from build123d import *

# Parameters (mm, degrees)
SKETCH003_W     = 170
SKETCH003_H     = 90
SKETCH003_W_2   = 160
SKETCH003_H_2   = 80
PAD_DEPTH       = 3
PAD001_DEPTH    = 3
PAD002_DEPTH    = 3
PAD003_DEPTH    = 3
PAD004_DEPTH    = 3
PAD005_DEPTH    = 10
PAD006_DEPTH    = 10
PAD007_DEPTH    = 24
SKETCH014_R     = 1.65
HOLE_DEPTH      = 30
SKETCH015_R     = 1.325
HOLE001_DEPTH   = 30
SKETCH016_R     = 1.325
HOLE002_DEPTH   = 30
SKETCH017_R     = 1.325
HOLE003_DEPTH   = 30
FILLET_R        = 0.3
FILLET001_R     = 0.3
FILLET002_R     = 0.3
FILLET003_R     = 0.3
FILLET004_R     = 0.3
FILLET005_R     = 0.3
FILLET006_R     = 0.3
FILLET007_R     = 0.3
FILLET008_R     = 0.3
FILLET009_R     = 0.3
SKETCH018_W     = 3.707428
SKETCH018_H     = 3.707435
PAD008_DEPTH    = 27
SKETCH019_W     = 4.325348
SKETCH019_H     = 3.769226
PAD009_DEPTH    = 27
SKETCH020_W     = 4.473305
SKETCH020_H     = 4.349049
PAD010_DEPTH    = 27
SKETCH021_W     = 3.413819
SKETCH021_H     = 3.638272
PAD011_DEPTH    = 27
SKETCH023_R     = 1.4
POCKET_DEPTH    = 30
SKETCH024_R     = 1.4
POCKET001_DEPTH = 30
SKETCH025_R     = 1.4
POCKET002_DEPTH = 30
SKETCH026_R     = 1.4
POCKET003_DEPTH = 30
SKETCH027_R     = 1.5
POCKET004_DEPTH = 5
CHAMFER_SIZE    = 1


with BuildPart() as part:
    # Sketch003 → Pad (new body)
    with BuildSketch(Plane.XY):
        Rectangle(SKETCH003_W, SKETCH003_H)
        Rectangle(SKETCH003_W_2, SKETCH003_H_2, mode=Mode.SUBTRACT)
    extrude(amount=PAD_DEPTH)

    # Sketch005 → Pad001 (join)
    with BuildSketch(Plane.XY):
        Polygon((-70, 45), (-75, 50), (-120, 50), (-120, 40), (-85, 5), (-85, 12), (-113, 40), (-95, 40), (-85, 30), (-85, 45), align=None)
    extrude(amount=PAD001_DEPTH)

    # Sketch007 → Pad002 (join)
    with BuildSketch(Plane.XY):
        Polygon((70, 45), (75, 50), (120, 50), (120, 40), (85, 5), (85, 12), (113, 40), (95, 40), (85, 30), (85, 45), align=None)
    extrude(amount=PAD002_DEPTH)

    # Sketch008 → Pad003 (join)
    with BuildSketch(Plane.XY):
        Polygon((70, -45), (75, -50), (120, -50), (120, -40), (85, -5), (85, -12), (113, -40), (95, -40), (85, -30), (85, -45), align=None)
    extrude(amount=PAD003_DEPTH)

    # Sketch009 → Pad004 (join)
    with BuildSketch(Plane.XY):
        Polygon((-70, -45), (-75, -50), (-115, -90), (-90, -115), (-90, -120), (-120, -120), (-120, -50), (-120, -40), (-85, -5), (-85, -12), (-113, -40), (-95, -40), (-85, -30), (-85, -45), align=None)
        Polygon((-115, -50), (-115, -83), (-82, -50), align=None, mode=Mode.SUBTRACT)
        Polygon((-115, -97), (-115, -115), (-97, -115), align=None, mode=Mode.SUBTRACT)
    extrude(amount=PAD004_DEPTH)

    # Sketch011 (on Face23 of Pad004) → Pad005 (join)
    with BuildSketch(Plane.XY.offset(3)):
        Polygon((-120, 50), (-120, 40), (-117, 40), (-117, 47), (-110, 47), (-110, 50), align=None)
    extrude(amount=PAD005_DEPTH)

    # Sketch012 (on Face22 of Pad005) → Pad006 (join)
    with BuildSketch(Plane.XY.offset(3)):
        Polygon((120, 50), (110, 50), (110, 47), (117, 47), (117, 40), (120, 40), align=None)
    extrude(amount=PAD006_DEPTH)

    # Sketch013 (on Face4 of Pad006) → Pad007 (join)
    with BuildSketch(Plane.XY.offset(3)):
        Polygon((-85, 45), (-85, 30), (-80, 30), (-80, 40), (-70, 40), (-70, 45), align=None)
        Polygon((85, 45), (85, 30), (80, 30), (80, 40), (70, 40), (70, 45), align=None)
        Polygon((85, -45), (85, -30), (80, -30), (80, -40), (70, -40), (70, -45), align=None)
        Polygon((-85, -45), (-85, -30), (-80, -30), (-80, -40), (-70, -40), (-70, -45), align=None)
    extrude(amount=PAD007_DEPTH)

    # Sketch014 (on Face80 of Pad007) → Hole (cut)
    with BuildSketch(Plane.XY.offset(27)):
        with Locations((-82.5, 42.5)):
            Circle(SKETCH014_R)
    extrude(amount=-HOLE_DEPTH, mode=Mode.SUBTRACT)

    # Sketch015 (on Face99 of Hole) → Hole001 (cut)
    with BuildSketch(Plane.XY.offset(27)):
        with Locations((-82.5, -42.5)):
            Circle(SKETCH015_R)
    extrude(amount=-HOLE001_DEPTH, mode=Mode.SUBTRACT)

    # Sketch016 (on Face84 of Hole001) → Hole002 (cut)
    with BuildSketch(Plane.XY.offset(27)):
        with Locations((82.5, 42.5)):
            Circle(SKETCH016_R)
    extrude(amount=-HOLE002_DEPTH, mode=Mode.SUBTRACT)

    # Sketch017 (on Face104 of Hole002) → Hole003 (cut)
    with BuildSketch(Plane.XY.offset(27)):
        with Locations((82.5, -42.5)):
            Circle(SKETCH017_R)
    extrude(amount=-HOLE003_DEPTH, mode=Mode.SUBTRACT)

    # Fillet
    fillet_edges = [part.edges().sort_by_distance(p)[0] for p in [
        (-115, -97, 1.5),
    ]]
    fillet(fillet_edges, radius=FILLET_R)

    # Fillet001
    fillet001_edges = [part.edges().sort_by_distance(p)[0] for p in [
        (-115, -115, 1.5),
    ]]
    fillet(fillet001_edges, radius=FILLET001_R)

    # Fillet002
    fillet002_edges = [part.edges().sort_by_distance(p)[0] for p in [
        (-97, -115, 1.5),
    ]]
    fillet(fillet002_edges, radius=FILLET002_R)

    # Fillet003
    fillet003_edges = [part.edges().sort_by_distance(p)[0] for p in [
        (-115, -90, 1.5),
    ]]
    fillet(fillet003_edges, radius=FILLET003_R)

    # Fillet004
    fillet004_edges = [part.edges().sort_by_distance(p)[0] for p in [
        (-115, -50, 1.5),
        (-115, -83, 1.5),
        (-82, -50, 1.5),
    ]]
    fillet(fillet004_edges, radius=FILLET004_R)

    # Fillet005
    fillet005_edges = [part.edges().sort_by_distance(p)[0] for p in [
        (-95, -40, 1.5),
        (-85, -12, 1.5),
        (-113, -40, 1.5),
    ]]
    fillet(fillet005_edges, radius=FILLET005_R)

    # Fillet006
    fillet006_edges = [part.edges().sort_by_distance(p)[0] for p in [
        (-117, 43.5, 3),
        (-113.5, 47, 3),
    ]]
    fillet(fillet006_edges, radius=FILLET006_R)

    # Fillet007
    fillet007_edges = [part.edges().sort_by_distance(p)[0] for p in [
        (-113, 40, 1.5),
        (-85, 12, 1.5),
    ]]
    fillet(fillet007_edges, radius=FILLET007_R)

    # Fillet008
    fillet008_edges = [part.edges().sort_by_distance(p)[0] for p in [
        (113.5, 47, 3),
        (117, 43.5, 3),
        (113, 40, 1.5),
        (85, 12, 1.5),
    ]]
    fillet(fillet008_edges, radius=FILLET008_R)

    # Fillet009
    fillet009_edges = [part.edges().sort_by_distance(p)[0] for p in [
        (113, -40, 1.5),
        (85, -12, 1.5),
    ]]
    fillet(fillet009_edges, radius=FILLET009_R)

    # Sketch018 (on Face81 of Fillet009) → Pad008 (join)
    with BuildSketch(Plane.XY.offset(27)):
        with Locations((82.542801, -42.437325)):
            Rectangle(SKETCH018_W, SKETCH018_H)
    extrude(amount=-PAD008_DEPTH)

    # Sketch019 (on Face37 of Pad008) → Pad009 (join)
    with BuildSketch(Plane.XY.offset(27)):
        with Locations((82.440964, 42.612553)):
            Rectangle(SKETCH019_W, SKETCH019_H)
    extrude(amount=-PAD009_DEPTH)

    # Sketch020 (on Face85 of Pad009) → Pad010 (join)
    with BuildSketch(Plane.XY.offset(27)):
        with Locations((-82.434589, 42.41842)):
            Rectangle(SKETCH020_W, SKETCH020_H)
    extrude(amount=-PAD010_DEPTH)

    # Sketch021 (on Face18 of Pad010) → Pad011 (join)
    with BuildSketch(Plane.XY.offset(27)):
        with Locations((-82.443809, -42.548483)):
            Rectangle(SKETCH021_W, SKETCH021_H)
    extrude(amount=-PAD011_DEPTH)

    # Sketch023 (on Face83 of Pad011) → Pocket (cut)
    with BuildSketch(Plane.XY.offset(27)):
        with Locations((-82.5, 42.5)):
            Circle(SKETCH023_R)
    extrude(amount=-POCKET_DEPTH, mode=Mode.SUBTRACT)

    # Sketch024 (on Face99 of Hole) → Pocket001 (cut)
    with BuildSketch(Plane.XY.offset(27)):
        with Locations((-82.5, -42.5)):
            Circle(SKETCH024_R)
    extrude(amount=-POCKET001_DEPTH, mode=Mode.SUBTRACT)

    # Sketch025 (on Face84 of Hole001) → Pocket002 (cut)
    with BuildSketch(Plane.XY.offset(27)):
        with Locations((82.5, 42.5)):
            Circle(SKETCH025_R)
    extrude(amount=-POCKET002_DEPTH, mode=Mode.SUBTRACT)

    # Sketch026 (on Face104 of Hole002) → Pocket003 (cut)
    with BuildSketch(Plane.XY.offset(27)):
        with Locations((82.5, -42.5)):
            Circle(SKETCH026_R)
    extrude(amount=-POCKET003_DEPTH, mode=Mode.SUBTRACT)

    # Sketch027 (on Face6 of Pocket003) → Pocket004 (cut)
    with BuildSketch(Plane.XY.offset(3)):
        with Locations((-115, -45)):
            Circle(SKETCH027_R)
        with Locations((115, -45)):
            Circle(SKETCH027_R)
    extrude(amount=-POCKET004_DEPTH, mode=Mode.SUBTRACT)

    # Chamfer
    chamfer_edges = [part.edges().sort_by_distance(p)[0] for p in [
        (-116.5, -45, 3),
        (113.5, -45, 3),
    ]]
    chamfer(chamfer_edges, length=CHAMFER_SIZE)


solid = part.part
Input: part model. Units: mm. Frame: model coordinates. A direction names the side the tool comes from. Coordinates: 2 decimals unless noted, no trailing zeros. Loops run counter-clockwise (first coordinate to the right, second up) from the corner with the lowest first, then second, coordinate; pieces in that order, holes last. Notation, with made-up numbers: (46, 32) - (57, 32) arc R25 cw to (57, 48) - close; hole circle Ø3 at (74, -29). An arc over 180 degrees is marked (long way). Answer in a Markdown table with one row per item. Add a question column.
Item 1: Access query for faces 1 (the flat face through (-70, -42, 15)), 2 (the flat face through (83, -30, 15)), 3 (the flat face through (117, 44, 8)), 4 (the flat face through (-103, 23, 1)), 5 (the flat face through (90, 35, 1)). Directions: +Z, -Z, +X, -X, +Y, -Y. A direction counts if a zero-diameter tool reaches every point of the face in a straight line with its end or side. Return the directions, or none.
Item 2: Section query A-A on z = 20.25. Return the cut outline in (x, y).
Item 3: Contact query for flat-ended pins moving along their axis: P1, Ø1.5, axis at x = 103.5, z = 1, coming from the -Y side; P2, Ø4, axis at x = -81.5, z = 13, coming from the +Y side; P3, Ø8, axis at y = -2, z = 9, coming from the +X side; P4, Ø1.5, axis at y = -70, z = 2, coming from the +X side. Output: stop coordinate, or through.
Item 4: Section query B-B on y = -77.5. Return the cut outline in (x, z).
Item 5: Line query: line 1 along Y through (x, z) = (82.5, 17); line 2 along X through (y, z) = (32, 2.25); line 3 along X through (y, z) = (37.5, 22). Output: solid intervals per line, ascending. Write a range as [from, to].
Item 6: Mould query, pull axis X, two halves, no side actions, for faces 6 (the flat face through (-103, -23, 1)), 7 (the flat face through (116, 47.3, 13)), 8 (the flat face through (-99, -26, 1)), 9 (the flat face through (85, -38, 15)). Classes: released by +X, released by -X, zero draft, split by the parting line, or undercut.
Recorded:
| question | item | result |
|---|---|---|
| 1 | face 1 | +Z, +Y, -Y |
| 1 | face 2 | +Z, +X, -X |
| 1 | face 3 | +Z, -Y |
| 1 | face 4 | +Z, -Z, -X |
| 1 | face 5 | +Z, -Z |
| 2 | outline | (-85, -45) - (-70, -45) - (-70, -40) - (-80, -40) - (-80, -30) - (-85, -30) - close; (-85, 30) - (-80, 30) - (-80, 40) - (-70, 40) - (-70, 45) - (-85, 45) - close; (70, -45) - (85, -45) - (85, -30) - (80, -30) - (80, -40) - (70, -40) - close; (70, 40) - (80, 40) - (80, 30) - (85, 30) - (85, 45) - (70, 45) - close; hole circle Ø2.8 at (-82.5, -42.5); hole circle Ø2.8 at (-82.5, 42.5); hole circle Ø2.8 at (82.5, -42.5); hole circle Ø2.8 at (82.5, 42.5) |
| 3 | P1 | y = -50 |
| 3 | P2 | y = 45 |
| 3 | P3 | through |
| 3 | P4 | x = -94.25 |
| 4 | outline | (-120, 0) - (-115, 0) - (-115, 3) - (-120, 3) - close; (-109.5, 0) - (-102.5, 0) - (-102.5, 3) - (-109.5, 3) - close |
| 5 | line 1 | [-45, -43.9], [-41.1, -30], [30, 41.1], [43.9, 45] |
| 5 | line 2 | [-112, -105], [-87, -80], [80, 87], [105, 112] |
| 5 | line 3 | [-85, -80], [80, 85] |
| 6 | face 6 | released by -X |
| 6 | face 7 | zero draft |
| 6 | face 8 | undercut |
| 6 | face 9 | released by +X |
